```python
from build123d import *

# Parameters (mm, degrees)
SKETCH1_W                     = 7.5
SKETCH1_H                     = 7.5
BOSS_EXTRUDE1_DEPTH           = 7
SKETCH2_W                     = 13
SKETCH2_H                     = 13
BOSS_EXTRUDE2_DEPTH           = 3.8
SKETCH3_W                     = 6
SKETCH3_H                     = 6
CUT_EXTRUDE1_DEPTH            = 15.182383439
SKETCH6_W                     = 12
SKETCH6_H                     = 12
CUT_EXTRUDE3_DEPTH            = 2.8
FILLET1_R                     = 0.5
BOSS_EXTRUDE3_REACH           = 16.182
FILLET4_R                     = 1.5
FILLET2_R                     = 1
TAP_DRILL_FOR_0_80_TAP1_D     = 1.19126
TAP_DRILL_FOR_0_80_TAP1_DEPTH = 7.11
TAP_DRILL_FOR_0_80_TAP1_TIP   = 0.357890611
FILLET5_R                     = 2.25
SKETCH16_W                    = 2.5
SKETCH16_H                    = 2
CUT_EXTRUDE4_DEPTH            = 0.835786
FILLET6_R                     = 1
SKETCH17_W                    = 2
SKETCH17_H                    = 2
SKETCH17_R                    = 0.375
BOSS_EXTRUDE4_DEPTH           = 3.8
FILLET7_R                     = 1


with BuildPart() as part:
    # Sketch1 → Boss-Extrude1 (new body)
    with BuildSketch(Plane(origin=(0, 0, 0), x_dir=(1, 0, 0), z_dir=(0, 1, 0))):
        Rectangle(SKETCH1_W, SKETCH1_H)
    extrude(amount=BOSS_EXTRUDE1_DEPTH)

    # Sketch2 → Boss-Extrude2 (add)
    with BuildSketch(Plane(origin=(0, 7, 0), x_dir=(1, 0, 0), z_dir=(0, 1, 0))):
        Rectangle(SKETCH2_W, SKETCH2_H)
    extrude(amount=BOSS_EXTRUDE2_DEPTH)

    # Sketch3 → Cut-Extrude1 (cut, through all)
    with BuildSketch(Plane.XZ):
        Rectangle(SKETCH3_W, SKETCH3_H)
    extrude(amount=-CUT_EXTRUDE1_DEPTH, mode=Mode.SUBTRACT)

    # Sketch6 → Cut-Extrude3 (cut)
    with BuildSketch(Plane(origin=(0, 10.8, 0), x_dir=(1, 0, 0), z_dir=(0, 1, 0))):
        Rectangle(SKETCH6_W, SKETCH6_H)
    extrude(amount=-CUT_EXTRUDE3_DEPTH, mode=Mode.SUBTRACT)

    # Fillet1
    fillet1_edges = [part.edges().sort_by_distance(p)[0] for p in [
        (6, 9.4, 6),
        (6, 9.4, -6),
        (-6, 9.4, -6),
        (-6, 9.4, 6),
    ]]
    fillet(fillet1_edges, radius=FILLET1_R)

    # Sketch12 → Boss-Extrude3 (add, up to next)
    with BuildSketch(Plane.XZ, mode=Mode.PRIVATE) as boss_extrude3_sk1:
        Polygon((3.75, -3.75), (4.633883476, -2.866116524), (3.75, -1.982233047), align=None)
    boss_extrude3_tool1 = extrude(boss_extrude3_sk1.sketch, amount=-BOSS_EXTRUDE3_REACH, mode=Mode.PRIVATE) - part.part
    # Sketch12 → Boss-Extrude3 (add, up to next)
    with BuildSketch(Plane.XZ, mode=Mode.PRIVATE) as boss_extrude3_sk2:
        Polygon((2.866116524, -4.633883476), (3.75, -3.75), (1.982233047, -3.75), align=None)
    boss_extrude3_tool2 = extrude(boss_extrude3_sk2.sketch, amount=-BOSS_EXTRUDE3_REACH, mode=Mode.PRIVATE) - part.part
    add(boss_extrude3_tool1.solids().sort_by_distance((4.044628, 0, -2.866117))[0])
    add(boss_extrude3_tool2.solids().sort_by_distance((2.866117, 0, -4.044628))[0])

    # Fillet4
    fillet4_edges = [part.edges().sort_by_distance(p)[0] for p in [
        (-3, 4, 3),
        (3, 4, 3),
        (-3, 4, -3),
        (3, 4, -3),
    ]]
    fillet(fillet4_edges, radius=FILLET4_R)

    # Fillet2
    fillet2_edges = [part.edges().sort_by_distance(p)[0] for p in [
        (3.75, 3.5, -1.982233047),
        (1.982233047, 3.5, -3.75),
    ]]
    fillet(fillet2_edges, radius=FILLET2_R)

    # Tap Drill for #0-80 Tap1
    with Locations(Plane(origin=(3.75, 0, -3.75), x_dir=(-0.7071067811865475, 0, -0.7071067811865477), z_dir=(0.7071067811865477, 0, -0.7071067811865475))):
        with Locations((0, 1.25), (0, 3.75)):
            Hole(TAP_DRILL_FOR_0_80_TAP1_D / 2, depth=TAP_DRILL_FOR_0_80_TAP1_DEPTH)
            with Locations((0, 0, -(TAP_DRILL_FOR_0_80_TAP1_DEPTH + TAP_DRILL_FOR_0_80_TAP1_TIP / 2))):  # 118° drill point
                Cone(0, TAP_DRILL_FOR_0_80_TAP1_D / 2, TAP_DRILL_FOR_0_80_TAP1_TIP, mode=Mode.SUBTRACT)

    # Fillet5
    fillet5_edges = [part.edges().sort_by_distance(p)[0] for p in [
        (3.75, 3.5, 3.75),
        (-3.75, 3.5, 3.75),
        (-3.75, 3.5, -3.75),
    ]]
    fillet(fillet5_edges, radius=FILLET5_R)

    # Sketch16 → Cut-Extrude4 (cut)
    with BuildSketch(Plane(origin=(3.75, 0, -3.75), x_dir=(-0.7071067811865474, 0, -0.7071067811865477), z_dir=(0.7071067811865477, 0, -0.7071067811865474))):
        with Locations((0, 6)):
            Rectangle(SKETCH16_W, SKETCH16_H)
    extrude(amount=-CUT_EXTRUDE4_DEPTH, mode=Mode.SUBTRACT)

    # Fillet6
    fillet6_edges = [part.edges().sort_by_distance(p)[0] for p in [
        (-6.5, 8.9, -6.5),
        (-6.5, 8.9, 6.5),
        (6.5, 8.9, 6.5),
        (6.5, 8.9, -6.5),
    ]]
    fillet(fillet6_edges, radius=FILLET6_R)

    # Sketch17 → Boss-Extrude4 (add)
    # profile 1 of 3: a face of its own
    with BuildSketch(Plane(origin=(0, 10.8, 0), x_dir=(1, 0, 0), z_dir=(0, 1, 0))):
        with Locations((-7.5, 0)):
            Rectangle(SKETCH17_W, SKETCH17_H)
        with Locations(Location((-7.5, 0, 0), (0, 0, 270))):
            Circle(SKETCH17_R, mode=Mode.SUBTRACT)
    # profile 2 of 3: a face of its own
    with BuildSketch(Plane(origin=(0, 10.8, 0), x_dir=(1, 0, 0), z_dir=(0, 1, 0))):
        with Locations((3.5, -7.5)):
            Rectangle(SKETCH17_W, SKETCH17_H)
        with Locations(Location((3.5, -7.5, 0), (0, 0, 270))):
            Circle(SKETCH17_R, mode=Mode.SUBTRACT)
    # profile 3 of 3: a face of its own
    with BuildSketch(Plane(origin=(0, 10.8, 0), x_dir=(1, 0, 0), z_dir=(0, 1, 0))):
        with Locations((3.5, 7.5)):
            Rectangle(SKETCH17_W, SKETCH17_H)
        with Locations(Location((3.5, 7.5, 0), (0, 0, 90))):
            Circle(SKETCH17_R, mode=Mode.SUBTRACT)
    extrude(amount=-BOSS_EXTRUDE4_DEPTH)

    # Fillet7
    fillet7_edges = [part.edges().sort_by_distance(p)[0] for p in [
        (-6.5, 8.9, 1),
        (-8.5, 8.9, 1),
        (-8.5, 8.9, -1),
        (-6.5, 8.9, -1),
        (2.5, 8.9, -6.5),
        (2.5, 8.9, -8.5),
        (4.5, 8.9, -8.5),
        (4.5, 8.9, -6.5),
        (2.5, 8.9, 6.5),
        (2.5, 8.9, 8.5),
        (4.5, 8.9, 8.5),
        (4.5, 8.9, 6.5),
    ]]
    fillet(fillet7_edges, radius=FILLET7_R - 0.0001)  # a hair under: the kernel refuses the full size


solid = part.part
```
Model file for the job. Use its own axes, mm. A direction names the side the tool comes from. Give positions to 0.01 mm unless a question says otherwise; leave off trailing zeros. Loops run counter-clockwise (first coordinate to the right, second up) from the corner with the lowest first, then second, coordinate; pieces in that order, holes last. Notation, with made-up numbers: (79, -36.5) -> (106, -36.5) arc R33 cw to (106, -1.5) -> close; hole circle Ø2 at (-18.5, 13). An arc over 180 degrees is marked (long way). Use CSV: the item, a comma, the result in double quotes. Start each with the question number.
1) Slice it at A-A on x = 0.25. Give the cut face in (y, z), plus the area to 3 significant figures.
2) Slice it at C-C on z = 2.75. Give the cut face in (x, y), plus the area to 3 significant figures.
3) Flat gauge pins, fed straight in: pin 1 Ø1.2 at (x, z) = (3.5, -3.5) entering from +Y; pin 2 Ø2.5 at (x, y) = (0.5, 3.5) entering from -Z; pin 3 Ø2 at (y, z) = (9, -5) entering from -X; pin 4 Ø1.4 at (y, z) = (8.5, 0.5) entering from -X. Where does each tip first touch, or does it go through?
4) Mould opens along X. For faces 6 (the cylindrical face through (-8.215, 8.873, -0.699)), 7 (the cylindrical face through (2.68, 3.78, -3.52)), 8 (the flat face through (3.75, 3, 0)) say: released by +X, released by -X, zero draft, split by the parting line, or undercut.
5) Slice it at D-D on y = 7.75. Give the number of separate pieces and of enclosed holes in the cut face, plus the area to 3 significant figures.
6) Slice it at B-B on z = -5. Give the cut face in (x, y).
7) Wall check: line 1 (X direction, y = 8.5, z = -2); line 2 (X direction, y = 8.65, z = 0) (3 decimals); line 3 (X direction, y = 7.5, z = 7.5) (3 decimals). Give the ranges that are in metal, low to high.
8) Tool access for faces 1 (the flat face through (3.7, 2.5, -3.8)), 2 (the flat face through (0, 9, 6)), 3 (the cylindrical face through (-3.11, 3.55, -3.07)), 4 (the flat face through (3, 4, 0)), 5 (the flat face through (-3.75, 3, 0)): list every direction of +Z, -Z, +X, -X, +Y, -Y with a clear straight run to the whole face (end or side of a thin tool).
Computed values:
1,outline,"(0, -3.75) -> (7, -3.75) -> (7, -6.5) -> (10.8, -6.5) -> (10.8, -6) -> (8, -6) -> (8, -3) -> (0, -3) -> close; (0, 3) -> (8, 3) -> (8, 6) -> (10.8, 6) -> (10.8, 6.5) -> (7, 6.5) -> (7, 3.75) -> (0, 3.75) -> close"
1,area,"20.3 mm^2"
2,outline,"(-6.5, 7) -> (-3.37, 7) -> (-3.37, 0) -> (-2.33, 0) -> (-2.33, 8) -> (-6, 8) -> (-6, 10.8) -> (-6.5, 10.8) -> close; (2.33, 0) -> (3.37, 0) -> (3.37, 7) -> (6.5, 7) -> (6.5, 10.8) -> (6, 10.8) -> (6, 8) -> (2.33, 8) -> close"
2,area,"25.7 mm^2"
3,pin 1,"stops at y = 8"
3,pin 2,"stops at z = -3.77"
3,pin 3,"stops at x = -6.5"
3,pin 4,"stops at x = -8.5"
4,face 6,"released by -X"
4,face 7,"undercut"
4,face 8,"released by +X"
5,separate pieces,"1"
5,enclosed holes,"4"
5,area,"145 mm^2"
6,outline,"(-6.5, 7) -> (6.5, 7) -> (6.5, 10.8) -> (6, 10.8) -> (6, 8) -> (-6, 8) -> (-6, 10.8) -> (-6.5, 10.8) -> close"
7,line 1,"x = -6.5 to -6, 6 to 6.5"
7,line 2,"x = -8.5 to -7.875, -7.125 to -6, 6 to 6.5"
7,line 3,"x = 2.5 to 3.125, 3.875 to 4.5"
8,face 1,"-Z, +X, -Y"
8,face 2,"+Y"
8,face 3,"-Z, -X, -Y"
8,face 4,"+Y, -Y"
8,face 5,"+Z, -Z, -X, -Y"
